Geometry: final body of the model. Coordinates: model frame, mm. Coordinates: 2 decimals unless noted, no trailing zeros. Write each loop counter-clockwise with the first axis right and the second up, starting at its lowest first coordinate (ties: lowest second). Pieces come first, ordered by that corner, then holes. Notation, with made-up numbers: (82.25, -34.75) -> (97.25, -34.75) arc R23 ccw to (97.25, -14.75) -> close; hole circle Ø11 at (43.5, 68). An arc over 180 degrees is marked (long way). One line per item, written item: value. Start each with the question number.
from build123d import *

# Parameters (mm, degrees)
SKETCH_1_W              = 48
SKETCH_1_H              = 10
EXTRUDE_1_DEPTH         = 5
HOLE_WIZARD_M4_1_D      = 3.3
HOLE_WIZARD_M4_2_D      = 3.3
CHAMFER_1_SIZE          = 0.2
HOLE_WIZARD_M4_3_REACH  = 50.518
HOLE_WIZARD_M4_3_BORE_R = 1.65
HOLE_WIZARD_M4_4_REACH  = 50.518
HOLE_WIZARD_M4_4_BORE_R = 1.65


with BuildPart() as part:
    # 草图1 → 凸台-拉伸1 (new, symmetric)
    with BuildSketch(Plane(origin=(0, 0, 0), x_dir=(1, 0, 0), z_dir=(0, 1, 0))):
        Rectangle(SKETCH_1_W, SKETCH_1_H)
    extrude(amount=EXTRUDE_1_DEPTH, both=True)

    # M4 螺纹孔1 (through all)
    with Locations(Plane(origin=(0, 5, 0), x_dir=(1, 0, 0), z_dir=(0, 1, 0))):
        with Locations((-8, 0), (8, 0)):
            Hole(HOLE_WIZARD_M4_1_D / 2)

    # M4 螺纹孔2 (through all)
    with Locations(Plane(origin=(0, 0, -5), x_dir=(-1, 0, 0), z_dir=(0, 0, -1))):
        with Locations((-16, 0), (16, 0)):
            Hole(HOLE_WIZARD_M4_2_D / 2)

    # 倒角1
    chamfer_1_edges = [part.edges().sort_by_distance(p)[0] for p in [
        (-24, 5, 0),
        (9.65, 5, 0),
        (9.65, -5, 0),
        (0, 5, 5),
        (-6.35, 5, 0),
        (-6.35, -5, 0),
        (-17.65, 0, -5),
        (-17.65, 0, 5),
        (14.35, 0, -5),
        (14.35, 0, 5),
        (24, 5, 0),
        (0, -5, 5),
        (-24, -5, 0),
        (0, -5, -5),
        (24, -5, 0),
        (24, 0, 5),
        (-24, 0, 5),
        (-24, 0, -5),
        (24, 0, -5),
        (0, 5, -5),
    ]]
    chamfer(chamfer_1_edges, length=CHAMFER_1_SIZE)

    # M4 螺纹孔3 bore → M4 螺纹孔3 (cut, up to next)
    with BuildSketch(Plane.ZY.offset(24), mode=Mode.PRIVATE) as hole_wizard_m4_3_sk1:
        Circle(HOLE_WIZARD_M4_3_BORE_R)
    hole_wizard_m4_3_tool1 = extrude(hole_wizard_m4_3_sk1.sketch, amount=-HOLE_WIZARD_M4_3_REACH, mode=Mode.PRIVATE) & part.part
    add(hole_wizard_m4_3_tool1.solids().sort_by_distance((-24, 0, 0))[0], mode=Mode.SUBTRACT)

    # M4 螺纹孔4 bore → M4 螺纹孔4 (cut, up to next)
    with BuildSketch(Plane(origin=(24, 0, 0), x_dir=(0, 0, -1), z_dir=(1, 0, 0)), mode=Mode.PRIVATE) as hole_wizard_m4_4_sk1:
        Circle(HOLE_WIZARD_M4_4_BORE_R)
    hole_wizard_m4_4_tool1 = extrude(hole_wizard_m4_4_sk1.sketch, amount=-HOLE_WIZARD_M4_4_REACH, mode=Mode.PRIVATE) & part.part
    add(hole_wizard_m4_4_tool1.solids().sort_by_distance((24, 0, 0))[0], mode=Mode.SUBTRACT)


solid = part.part
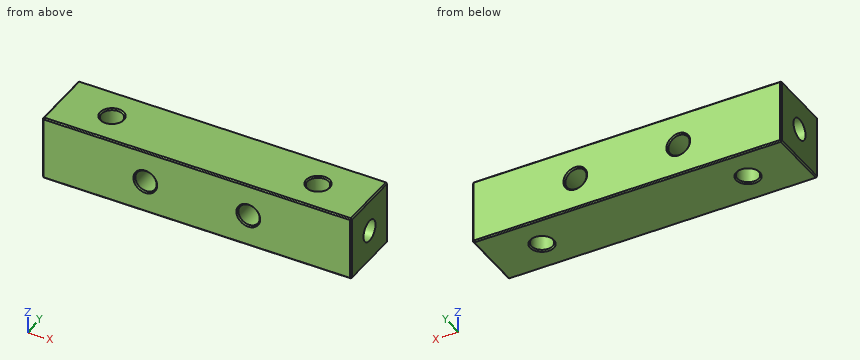
Q1. Cut plane B-B on x = 21.5. Output: boundary loops of the cut face in (y, z).
Q2. Cut plane C-C on x = 8. Output: boundary loops of the cut face in (y, z), and give its area (3 significant figures).
Q3. Line query: L1, parallel to X at y = -2.5, z = 0; L2, parallel to Y at x = 18, z = 0; L3, parallel to X at y = 0.5, z = -1.75. Output: solid intervals per line, ascending. Write a range as from..to.
Q4. Cut plane D-D on z = 4. Output: boundary loops of the cut face in (x, y), and give its area (3 significant figures).
Q5. Cut plane A-A on z = 0. Count the separate pieces of the cut face and the enclosed holes in it, and give its area (3 significant figures).
Q6. First-contact query: P1, Ø2, axis at x = 8, z = 0, coming from the +Y side. Flat tip, straight axial feed; report the tip coordinate or a pass-through.
Solution:
1. outline: (-5, -4.8) -> (-4.8, -5) -> (4.8, -5) -> (5, -4.8) -> (5, 4.8) -> (4.8, 5) -> (-4.8, 5) -> (-5, 4.8) -> close; hole circle Ø3.3 at (0, 0)
2. outline: (-5, -4.8) -> (-4.8, -5) -> (4.8, -5) -> (5, -4.8) -> (5, -1.85) -> (4.8, -1.65) -> (-4.8, -1.65) -> (-5, -1.85) -> close; (-5, 1.85) -> (-4.8, 1.65) -> (4.8, 1.65) -> (5, 1.85) -> (5, 4.8) -> (4.8, 5) -> (-4.8, 5) -> (-5, 4.8) -> close
2. area: 66.8 mm²
3. L1: -24..-9.65, -6.35..6.35, 9.65..24
3. L2: -5..-1.65, 1.65..5
3. L3: -24..-17.57, -14.43..14.43, 17.57..24
4. outline: (-24, -4.8) -> (-23.8, -5) -> (23.8, -5) -> (24, -4.8) -> (24, 4.8) -> (23.8, 5) -> (-23.8, 5) -> (-24, 4.8) -> close; hole circle Ø3.3 at (-16, 0); hole circle Ø3.3 at (16, 0)
4. area: 463 mm²
5. separate pieces: 3
5. enclosed holes: 0
5. area: 352 mm²
6. P1: through
